Could you check a few things on this model? Use its own coordinates, in mm. A direction names the side the tool comes from. Round coordinates to 2 decimals unless told otherwise and drop trailing zeros. Write each loop counter-clockwise with the first axis right and the second up, starting at its lowest first coordinate (ties: lowest second). Pieces come first, ordered by that corner, then holes. Notation, with made-up numbers: M 63.5,57 L 96.5,57 A28 ccw 96.5,81 Z; hole C -32,20 d6. An arc over 180 degrees is marked long. One line per item, written item: value. Start each with the question number.
(1) Thinking about a two-plate mould opening in X: for faces 3 (the face through (17, -2, -40.25)), 4 (the face through (-4, -2, 0)), 5 (the face through (-27, -3, -1)), which applies, released by +X, released by -X, zero draft, split by the parting line, or undercut?
(2) I'm going to push flat-ended pins straight in: pin 1 Ø2.5 at (x, z) = (-23.5, -4) entering from +Y; pin 2 Ø4 at (x, z) = (20, -10.75) entering from +Y. Where does each tip first touch, or does it pass through?
(3) I want a section at A-A on z = -4. Please give me the cut outline in (x, y).
(4) Which directions (+Z, -Z, +X, -X, +Y, -Y) give clear straight access to the entire face, cutting with the end or side of a thin tool? Please do faces 1 (the face through (0, 0, -23)), 2 (the face through (-3.5, -2, -11)).
(5) I want a section at B-B on x = 14. Please give me the cut outline in (y, z), and give its area (3 significant figures).
(6) I want a section at D-D on x = -8.5. Please give me the cut outline in (y, z).
(7) If I drill on L1, parallel to Z at x = -8.5, y = -2.3; L2, parallel to X at y = -3, z = -10.75; L3, parallel to X at y = -3.55, z = -17.5, over which ranges is the centre line in solid material (lowest first)?
(8) I want a section at C-C on z = -10.75. Please give me the cut outline in (x, y).
```python
from build123d import *

# Parameters (mm, degrees)
BASE_SKETCH_W               = 55
BASE_SKETCH_H               = 45
BASE_EXTRUDE_DEPTH          = 5
MOSFET_MOUNTING_HOLES_D     = 1.6
MOUNTING_HOLES_D            = 3.6576
MOUNTING_HOLES_CSINK_D      = 7.0866
MOUNTING_HOLES_CSINK_ANGLE  = 82
PIN_RELIEF_SKETCH_W         = 12
PIN_RELIEF_SKETCH_H         = 12
CUT_TERMAL_PIN_RELIEF_DEPTH = 53.974050251
FILLET1_R                   = 10
FILLET2_R                   = 2.5
FILLET3_R                   = 1


with BuildPart() as part:
    # Base Sketch → Base Extrude (new body)
    with BuildSketch(Plane(origin=(0, 0, 0), x_dir=(1, 0, 0), z_dir=(0, 1, 0))):
        with Locations((0, 22.5)):
            Rectangle(BASE_SKETCH_W, BASE_SKETCH_H)
    extrude(amount=-BASE_EXTRUDE_DEPTH)

    # Mosfet Mounting Holes (through all)
    with Locations(Plane(origin=(0, 0, 0), x_dir=(1, 0, 0), z_dir=(0, 1, 0))):
        with Locations((-23.5, 4), (-23.5, 17.5), (-8.5, 27.5), (-8.5, 41)):
            Hole(MOSFET_MOUNTING_HOLES_D / 2)

    # Mounting Holes (through all)
    with Locations(Plane(origin=(0, 0, 0), x_dir=(1, 0, 0), z_dir=(0, 1, 0))):
        with Locations((-20, 34.25), (20, 10.75)):
            CounterSinkHole(MOUNTING_HOLES_D / 2, MOUNTING_HOLES_CSINK_D / 2, counter_sink_angle=MOUNTING_HOLES_CSINK_ANGLE)

    # Pin Relief Sketch → Cut Termal Pin Relief (cut, through all)
    with BuildSketch(Plane(origin=(0, 0, 0), x_dir=(1, 0, 0), z_dir=(0, 1, 0))):
        with Locations((2.5, 10.75)):
            Rectangle(PIN_RELIEF_SKETCH_W, PIN_RELIEF_SKETCH_H)
        with Locations((17.5, 34.25)):
            Rectangle(PIN_RELIEF_SKETCH_W, PIN_RELIEF_SKETCH_H)
    extrude(amount=-CUT_TERMAL_PIN_RELIEF_DEPTH, mode=Mode.SUBTRACT)

    # Fillet1
    fillet1_edges = [part.edges().sort_by_distance(p)[0] for p in [
        (-27.5, -2.5, -45),
        (27.5, -2.5, 0),
    ]]
    fillet(fillet1_edges, radius=FILLET1_R)

    # Fillet2
    fillet2_edges = [part.edges().sort_by_distance(p)[0] for p in [
        (27.5, -2.5, -45),
        (-27.5, -2.5, 0),
    ]]
    fillet(fillet2_edges, radius=FILLET2_R)

    # Fillet3
    fillet3_edges = [part.edges().sort_by_distance(p)[0] for p in [
        (-3.5, -2.5, -4.75),
        (-3.5, -2.5, -16.75),
        (8.5, -2.5, -16.75),
        (8.5, -2.5, -4.75),
        (11.5, -2.5, -28.25),
        (11.5, -2.5, -40.25),
        (23.5, -2.5, -40.25),
        (23.5, -2.5, -28.25),
    ]]
    fillet(fillet3_edges, radius=FILLET3_R)


solid = part.part
```
Found:
1. face 3: undercut
1. face 4: zero draft
1. face 5: released by -X
2. pin 1: stops at y = 0
2. pin 2: stops at y = -1.78
3. outline: M -27.5,-5 L -24.3,-5 L -24.3,0 L -27.5,0 Z; M -22.7,-5 L 25.5,-5 L 25.5,0 L -22.7,0 Z
4. face 1: +Z, -Z, +X, -X, +Y
4. face 2: +Y, -Y
5. outline: M -5,-45 L 0,-45 L 0,-40.25 L -5,-40.25 Z; M -5,-28.25 L 0,-28.25 L 0,0 L -5,0 Z
5. area: 165 mm²
6. outline: M -5,-45 L 0,-45 L 0,-41.8 L -5,-41.8 Z; M -5,-40.2 L 0,-40.2 L 0,-28.3 L -5,-28.3 Z; M -5,-26.7 L 0,-26.7 L 0,0 L -5,0 Z
7. L1: z = -45 to -41.8, -40.2 to -28.3, -26.7 to 0
7. L2: x = -27.5 to -3.5, 8.5 to 18.17, 21.83 to 27.5
7. L3: x = -27.5 to -24.3, -22.7 to 27.5
8. outline: M -27.5,-5 L -3.5,-5 L -3.5,0 L -27.5,0 Z; M 8.5,-5 L 18.17,-5 L 18.17,-1.97 L 16.46,0 L 8.5,0 Z; M 21.83,-5 L 27.5,-5 L 27.5,0 L 23.54,0 L 21.83,-1.97 Z
